```python
from build123d import *

# Parameters (mm, degrees)
SKETCH1_R           = 50
BOSS_EXTRUDE1_DEPTH = 10
SKETCH2_R           = 15
BOSS_EXTRUDE2_DEPTH = 20
SKETCH5_R           = 8
CUT_EXTRUDE2_DEPTH  = 5
SKETCH6_R           = 6
CUT_EXTRUDE3_DEPTH  = 76
SKETCH7_R           = 1.75
CUT_EXTRUDE4_DEPTH  = 77.811457479
SKETCH8_R           = 2.25
CUT_EXTRUDE5_DEPTH  = 77.811457479


with BuildPart() as part:
    # Sketch1 → Boss-Extrude1 (new body)
    with BuildSketch(Plane.XY):
        Circle(SKETCH1_R)
    extrude(amount=BOSS_EXTRUDE1_DEPTH)

    # Sketch2 → Boss-Extrude2 (add)
    with BuildSketch(Plane.XY.offset(10)):
        Circle(SKETCH2_R)
    extrude(amount=BOSS_EXTRUDE2_DEPTH)

    # Sketch5 → Cut-Extrude2 (cut)
    with BuildSketch(Plane.XY.offset(30)):
        Circle(SKETCH5_R)
    extrude(amount=-CUT_EXTRUDE2_DEPTH, mode=Mode.SUBTRACT)

    # Sketch6 → Cut-Extrude3 (cut, through all)
    with BuildSketch(Plane.XY.offset(25)):
        Circle(SKETCH6_R)
    extrude(amount=-CUT_EXTRUDE3_DEPTH, mode=Mode.SUBTRACT)

    # Sketch7 → Cut-Extrude4 (cut, through all)
    with BuildSketch(Plane(origin=(0, 0, 0), x_dir=(-1, 0, 0), z_dir=(0, 0, -1))):
        with Locations((-28.25, 29)):
            Circle(SKETCH7_R)
        with Locations(Location((28.25, 29, 0), (0, 0, 180))):
            Circle(SKETCH7_R)
        with Locations((28.25, -29)):
            Circle(SKETCH7_R)
        with Locations(Location((-28.25, -29, 0), (0, 0, 180))):
            Circle(SKETCH7_R)
    extrude(amount=-CUT_EXTRUDE4_DEPTH, mode=Mode.SUBTRACT)

    # Sketch8 → Cut-Extrude5 (cut, through all)
    with BuildSketch(Plane(origin=(0, 0, 0), x_dir=(-1, 0, 0), z_dir=(0, 0, -1))):
        with Locations((0, 19)):
            Circle(SKETCH8_R)
        with Locations(Location((0, -19, 0), (0, 0, 180))):
            Circle(SKETCH8_R)
    extrude(amount=-CUT_EXTRUDE5_DEPTH, mode=Mode.SUBTRACT)


solid = part.part
```
The model under review builds one solid part; all positions refer to its coordinate system, in mm. A direction names the side the tool comes from. Give positions to 0.01 mm unless a question says otherwise; leave off trailing zeros. Order: outer loops, then holes, each group sorted by start corner. A loop starts at its lowest first (then second) coordinate and runs counter-clockwise, first axis right, second up. Notation, with made-up numbers: (-2, 65) - (2, 65) arc R25 ccw to (2, 104) - close; hole circle Ø10 at (-27.75, 87.25). An arc over 180 degrees is marked (long way). Use CSV: the item, a comma, the result in double quotes. Start each with the question number.
Q1. We need section C-C, the plane x = 28.25. Write out the cut boundary in (y, z).
Q2. We need section D-D, the plane y = -29. Write out the cut boundary in (x, z), and give its area (3 significant figures).
Q3. Clearance check with flat-ended pins moving along their axes: pin 1 Ø10 at (y, z) = (13, 10.5) entering from +X; pin 2 Ø12 at (x, y) = (25, 29) entering from +Z; pin 3 Ø4 at (y, z) = (25, 6.5) entering from -X. State where each tip first meets the part, or that it passes through.
Q4. The part is to be moulded in two halves that separate along Y. For faces 3 (the flat face through (-1, -10, 0)), 4 (the cylindrical face through (-14.985, 0.66, 19.86)), 5 (the cylindrical face through (-1.73, -7.81, 27.54)), 6 (the cylindrical face through (26.5, -29.08, 4.93)), say which applies: +Y half, -Y half, draft (parallel to the pull), parting line (faces both ways), or undercut.
Q5. Tool access review of faces 1 (the flat face through (-2, 6, 25)), 2 (the cylindrical face through (-26.86, -30.06, 4.93)): name each direction out of +Z, -Z, +X, -X, +Y, -Y from which nothing blocks a thin tool from reaching the whole face with its end or side.
Q6. We need section A-A, the plane y = 0. Write out the cut boundary in (x, z).
Q7. To check wall thickness, follow line 1 along Y through (x, z) = (-28.25, 7); line 2 along Z through (x, y) = (45, -15); line 3 along Y through (x, z) = (0, 19.75). State the ranges of each line that lie inside material, in increasing order. Write a range as [from, to].
Q8. We need section B-B, the plane x = 0. Write out the cut boundary in (y, z), and give its area (3 significant figures).
Outcome:
1,outline,"(-41.25, 0) - (-30.75, 0) - (-30.75, 10) - (-41.25, 10) - close; (-27.25, 0) - (27.25, 0) - (27.25, 10) - (-27.25, 10) - close; (30.75, 0) - (41.25, 0) - (41.25, 10) - (30.75, 10) - close"
2,outline,"(-40.73, 0) - (-30, 0) - (-30, 10) - (-40.73, 10) - close; (-26.5, 0) - (26.5, 0) - (26.5, 10) - (-26.5, 10) - close; (30, 0) - (40.73, 0) - (40.73, 10) - (30, 10) - close"
2,area,"745 mm^2"
3,pin 1,"stops at x = 49.35"
3,pin 2,"stops at z = 10"
3,pin 3,"stops at x = -44.4"
4,face 3,"draft"
4,face 4,"parting line"
4,face 5,"undercut"
4,face 6,"undercut"
5,face 1,"+Z"
5,face 2,"+Z, -Z"
6,outline,"(-50, 0) - (-6, 0) - (-6, 25) - (-8, 25) - (-8, 30) - (-15, 30) - (-15, 10) - (-50, 10) - close; (6, 0) - (50, 0) - (50, 10) - (15, 10) - (15, 30) - (8, 30) - (8, 25) - (6, 25) - close"
7,line 1,"y = [-41.25, -30.75], [-27.25, 27.25], [30.75, 41.25]"
7,line 2,"z = [0, 10]"
7,line 3,"y = [-15, -6], [6, 15]"
8,outline,"(-50, 0) - (-21.25, 0) - (-21.25, 10) - (-50, 10) - close; (-16.75, 0) - (-6, 0) - (-6, 25) - (-8, 25) - (-8, 30) - (-15, 30) - (-15, 10) - (-16.75, 10) - close; (6, 0) - (16.75, 0) - (16.75, 10) - (15, 10) - (15, 30) - (8, 30) - (8, 25) - (6, 25) - close; (21.25, 0) - (50, 0) - (50, 10) - (21.25, 10) - close"
8,area,"1,130 mm^2"
